Build history of the part. All positions in model axes, mm. A direction names the side the tool comes from. Coordinates: 2 decimals unless noted, no trailing zeros. Order: outer loops, then holes, each group sorted by start corner. A loop starts at its lowest first (then second) coordinate and runs counter-clockwise, first axis right, second up. Notation, with made-up numbers: (85, 28) -> (97, 28) arc R15 ccw to (97, 50) -> close; hole circle Ø10 at (10.5, 64.5). An arc over 180 degrees is marked (long way). Write each question's results on one line, items separated by ' | '.
from build123d import *

# Parameters (mm, degrees)
F0_W           = 150
F0_H           = 70
F1_DEPTH       = 25
F3_D           = 11
F3_CBORE_D     = 17.25
F3_CBORE_DEPTH = 10
F4_SIZE        = 5
F5_SIZE        = 5
F6_W           = 30
F6_H           = 25
F7_DEPTH       = 25
F9_D           = 10


with BuildPart() as f1:
    # F0 (on Top) → F1 (new body)
    with BuildSketch(Plane.XY):
        Rectangle(F0_W, F0_H)
    extrude(amount=F1_DEPTH)

    # F3 (through all)
    with Locations(Plane(origin=(0, 0, 0), x_dir=(1, 0, 0), z_dir=(0, 0, -1))):
        with Locations((-50, -25), (-50, 25), (50, 25), (50, -25)):
            CounterBoreHole(F3_D / 2, F3_CBORE_D / 2, F3_CBORE_DEPTH)

    # F4
    f4_edges = [f1.edges().sort_by_distance(p)[0] for p in [
        (-75, 35, 12.5),
        (-75, -35, 12.5),
    ]]
    chamfer(f4_edges, length=F4_SIZE)

    # F5
    f5_edges = [f1.edges().sort_by_distance(p)[0] for p in [
        (75, 35, 12.5),
        (75, -35, 12.5),
    ]]
    chamfer(f5_edges, length=F5_SIZE)

    # F6 (on face) → F7 (cut)
    with BuildSketch(Plane(origin=(0, 0, 0), x_dir=(1, 0, 0), z_dir=(0, 0, -1))):
        with Locations((0, -32.5)):
            Rectangle(F6_W, F6_H)
    extrude(amount=-F7_DEPTH, mode=Mode.SUBTRACT)

    # F9 (through all)
    with Locations(Plane.XY.offset(25)):
        with Locations((0, 0)):
            Hole(F9_D / 2)


solid = f1.part
Item 1: Slice it at D-D, the plane x = -50. List the corners of the cut face in (y, z) (3 decimals), and give its area (4 significant figures).
Answer:
outline: (-35, 0) -> (-33.625, 0) -> (-33.625, 10) -> (-30.5, 10) -> (-30.5, 25) -> (-35, 25) -> close; (-19.5, 10) -> (-16.375, 10) -> (-16.375, 0) -> (16.375, 0) -> (16.375, 10) -> (19.5, 10) -> (19.5, 25) -> (-19.5, 25) -> close; (30.5, 10) -> (33.625, 10) -> (33.625, 0) -> (35, 0) -> (35, 25) -> (30.5, 25) -> close | area: 1,075 mm^2
Item 2: Pull direction Y, two halves, no side cores. Call faces 1 (the flat face through (0, 20, 12)), 2 (the cylindrical face through (-44.505, -25.242, 17.605)), 3 (the flat face through (75, 0, 12)): released by +Y, released by -Y, zero draft, split by the parting line, or undercut.
Answer:
face 1: released by +Y | face 2: undercut | face 3: zero draft
Item 3: Slice it at A-A, the plane y = -25. List the corners of the cut face in (x, z) (3 decimals).
Answer:
outline: (-75, 0) -> (-58.625, 0) -> (-58.625, 10) -> (-55.5, 10) -> (-55.5, 25) -> (-75, 25) -> close; (-44.5, 10) -> (-41.375, 10) -> (-41.375, 0) -> (41.375, 0) -> (41.375, 10) -> (44.5, 10) -> (44.5, 25) -> (-44.5, 25) -> close; (55.5, 10) -> (58.625, 10) -> (58.625, 0) -> (75, 0) -> (75, 25) -> (55.5, 25) -> close
Item 4: Drill centre lines: line 1 (X direction, y = 25, z = 21.75); line 2 (Y direction, x = -50, z = 17.25); line 3 (Y direction, x = 50, z = 7.5) (3 decimals). Where is each one in solid material? Low to high. Write a range as from..to.
Answer:
line 1: x = -75..-55.5, -44.5..-15, 15..44.5, 55.5..75 | line 2: y = -35..-30.5, -19.5..19.5, 30.5..35 | line 3: y = -35..-33.625, -16.375..16.375, 33.625..35
Item 5: Slice it at C-C, the plane z = 15.5. List the corners of the cut face in (x, y), and give its area (3 significant figures).
Answer:
outline: (-75, -30) -> (-70, -35) -> (70, -35) -> (75, -30) -> (75, 30) -> (70, 35) -> (15, 35) -> (15, 20) -> (-15, 20) -> (-15, 35) -> (-70, 35) -> (-75, 30) -> close; hole circle Ø11 at (-50, -25); hole circle Ø11 at (-50, 25); hole circle Ø10 at (0, 0); hole circle Ø11 at (50, -25); hole circle Ø11 at (50, 25) | area: 9,540 mm^2
Item 6: Pin check, flat tips, straight feed: pin 1 (4 mm diameter, centred on x = 10.5, z = 14.5, fed in from +Y); pin 2 (5 mm diameter, centred on x = -46.5, y = 23.5, fed in from -Z). Stop position of each tip, or through.
Answer:
pin 1: stops at y = 20 | pin 2: stops at z = 10
Item 7: Slice it at B-B, the plane y = 25. List the corners of the cut face in (x, z) (3 decimals), and give its area (4 significant figures).
Answer:
outline: (-75, 0) -> (-58.625, 0) -> (-58.625, 10) -> (-55.5, 10) -> (-55.5, 25) -> (-75, 25) -> close; (-44.5, 10) -> (-41.375, 10) -> (-41.375, 0) -> (-15, 0) -> (-15, 25) -> (-44.5, 25) -> close; (15, 0) -> (41.375, 0) -> (41.375, 10) -> (44.5, 10) -> (44.5, 25) -> (15, 25) -> close; (55.5, 10) -> (58.625, 10) -> (58.625, 0) -> (75, 0) -> (75, 25) -> (55.5, 25) -> close | area: 2,325 mm^2
Item 8: Tool access for faces 4 (the cylindrical face through (53.98, -17.35, 4.93)), 5 (the cylindrical face through (1.08, -4.88, 12.32)), 6 (the flat face through (-15, 28, 12)): list every direction of +Z, -Z, +X, -X, +Y, -Y with a clear straight run to the whole face (end or side of a thin tool).
Answer:
face 4: -Z | face 5: +Z, -Z | face 6: +Z, -Z, +Y
